Source: CAD feature listing. Evaluate the final solid. Frame: model axes, mm. Face numbers are marked on the shaded views. Coordinates: 2 decimals unless noted, no trailing zeros. Order: outer loops, then holes, each group sorted by start corner. A loop starts at its lowest first (then second) coordinate and runs counter-clockwise, first axis right, second up. Notation, with made-up numbers: (27.25, 55.25) -> (60.25, 55.25) arc R16 ccw to (60.25, 81.25) -> close; hole circle Ø10 at (-13.75, 73.25). An arc over 180 degrees is marked (long way). Write each question's results on one line, items separated by ' | '. Start each with the question number.
from build123d import *

# Parameters (mm, degrees)
IZIM1_R                     = 37.5
Y_KSEKLIK_EKSTR_ZYON1_DEPTH = 30


with BuildPart() as part:
    # Çizim1 → Yükseklik-Ekstrüzyon1 (new body)
    with BuildSketch(Plane(origin=(0, 0, 0), x_dir=(1, 0, 0), z_dir=(0, 1, 0))):
        with Locations(Location((0, 0, 0), (0, 0, 270))):
            Circle(IZIM1_R)
        with BuildLine():
            ThreePointArc((-18.874079265, -29.690864233), (-30.468569301, -17.591036688), (-35.150082319, -1.5))
            Line((-35.150082319, -1.5), (-9.196399109, -1.5))
            ThreePointArc((-9.196399109, -1.5), (-8.069561167, -4.658963312), (-5.89723766, -7.214315252))
            Line((-5.89723766, -7.214315252), (-18.874079265, -29.690864233))
        make_face(mode=Mode.SUBTRACT)
        with BuildLine():
            Line((3.299161449, -8.714315252), (16.276003054, -31.190864233))
            ThreePointArc((16.276003054, -31.190864233), (0, -35.182073376), (-16.276003054, -31.190864233))
            Line((-16.276003054, -31.190864233), (-3.299161449, -8.714315252))
            ThreePointArc((-3.299161449, -8.714315252), (0, -9.317926624), (3.299161449, -8.714315252))
        make_face(mode=Mode.SUBTRACT)
        with BuildLine():
            Line((9.196399109, -1.5), (35.150082319, -1.5))
            ThreePointArc((35.150082319, -1.5), (30.468569301, -17.591036688), (18.874079265, -29.690864233))
            Line((18.874079265, -29.690864233), (5.89723766, -7.214315252))
            ThreePointArc((5.89723766, -7.214315252), (8.069561167, -4.658963312), (9.196399109, -1.5))
        make_face(mode=Mode.SUBTRACT)
        with BuildLine():
            ThreePointArc((-35.150082319, 1.5), (-30.468569301, 17.591036688), (-18.874079265, 29.690864233))
            Line((-18.874079265, 29.690864233), (-5.89723766, 7.214315252))
            ThreePointArc((-5.89723766, 7.214315252), (-8.069561167, 4.658963312), (-9.196399109, 1.5))
            Line((-9.196399109, 1.5), (-35.150082319, 1.5))
        make_face(mode=Mode.SUBTRACT)
        with BuildLine():
            Line((6.34428877, -4), (-6.34428877, -4))
            ThreePointArc((-6.34428877, -4), (0, 7.5), (6.34428877, -4))
        make_face(mode=Mode.SUBTRACT)
        with BuildLine():
            Line((5.89723766, 7.214315252), (18.874079265, 29.690864233))
            ThreePointArc((18.874079265, 29.690864233), (30.468569301, 17.591036688), (35.150082319, 1.5))
            Line((35.150082319, 1.5), (9.196399109, 1.5))
            ThreePointArc((9.196399109, 1.5), (8.069561167, 4.658963312), (5.89723766, 7.214315252))
        make_face(mode=Mode.SUBTRACT)
        with BuildLine():
            Line((-3.299161449, 8.714315252), (-16.276003054, 31.190864233))
            ThreePointArc((-16.276003054, 31.190864233), (0, 35.182073376), (16.276003054, 31.190864233))
            Line((16.276003054, 31.190864233), (3.299161449, 8.714315252))
            ThreePointArc((3.299161449, 8.714315252), (0, 9.317926624), (-3.299161449, 8.714315252))
        make_face(mode=Mode.SUBTRACT)
    extrude(amount=Y_KSEKLIK_EKSTR_ZYON1_DEPTH)


solid = part.part
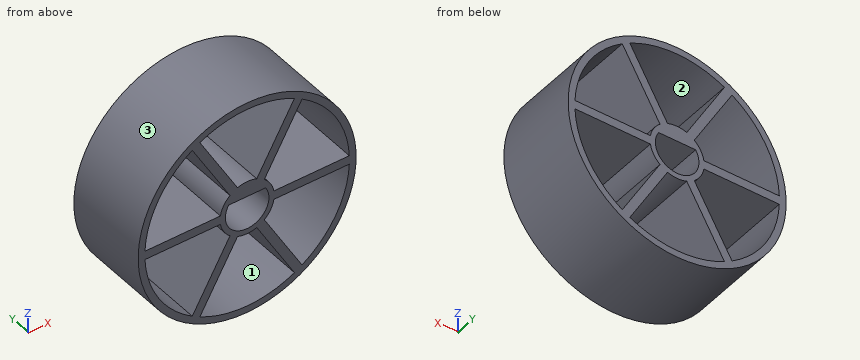
(1) First-contact query: P1, Ø1, axis at y = 19, z = -3, coming from the +X side; P2, Ø1, axis at y = 26.5, z = -24.5, coming from the +X side; P3, Ø12, axis at x = 0, z = 0, coming from the -Y side; P4, Ø8, axis at y = 7.5, z = 30, coming from the +X side. Flat tips, straight axial feed; report the tip coordinate or a pass-through.
(2) Section B-B on y = 20.5. Return the cut outline in (x, z).
(3) Draft query along X for the marked faces 1, 2 and 3. Return one class per face: released by +X, released by -X, zero draft, split by the parting line, or undercut.
(4) Section C-C on x = 0. Return the cut outline in (y, z), then the cut area to 3 significant figures.
(5) Section A-A on z = 0. Return the cut outline in (x, y).
(6) Section D-D on x = -32. Return the cut outline in (y, z), then the cut area to 3 significant figures.
(7) Line query: L1, parallel to X at y = 16, z = 0; L2, parallel to Z at x = -25, y = 20; L3, parallel to Z at x = -15, y = 18. Output: solid intervals per line, ascending.
Results list:
1) P1: stops at x = 37.42 | P2: stops at x = 28.81 | P3: stops at y = 0 | P4: stops at x = 27.02
2) outline: circle Ø75 at (0, 0); hole (-35.15, -1.5) arc R35.18 ccw to (-18.87, -29.69) -> (-5.9, -7.21) arc R9.32 cw to (-9.2, -1.5) -> close; hole (-35.15, 1.5) -> (-9.2, 1.5) arc R9.32 cw to (-5.9, 7.21) -> (-18.87, 29.69) arc R35.18 ccw to start; hole (-16.28, -31.19) arc R35.18 ccw to (16.28, -31.19) -> (3.3, -8.71) arc R9.32 cw to (-3.3, -8.71) -> close; hole (-16.28, 31.19) -> (-3.3, 8.71) arc R9.32 cw to (3.3, 8.71) -> (16.28, 31.19) arc R35.18 ccw to start; hole (-6.34, 4) arc R7.5 ccw (long way) to (6.34, 4) -> close; hole (5.9, -7.21) -> (18.87, -29.69) arc R35.18 ccw to (35.15, -1.5) -> (9.2, -1.5) arc R9.32 cw to start; hole (5.9, 7.21) arc R9.32 cw to (9.2, 1.5) -> (35.15, 1.5) arc R35.18 ccw to (18.87, 29.69) -> close
3) face 1: undercut | face 2: undercut | face 3: split by the parting line
4) outline: (0, -37.5) -> (30, -37.5) -> (30, -35.18) -> (0, -35.18) -> close; (0, -9.32) -> (30, -9.32) -> (30, -7.5) -> (0, -7.5) -> close; (0, 4) -> (30, 4) -> (30, 9.32) -> (0, 9.32) -> close; (0, 35.18) -> (30, 35.18) -> (30, 37.5) -> (0, 37.5) -> close | area: 353 mm²
5) outline: (-37.5, 0) -> (-7.5, 0) -> (-7.5, 30) -> (-37.5, 30) -> close; (7.5, 0) -> (37.5, 0) -> (37.5, 30) -> (7.5, 30) -> close
6) outline: (0, -19.55) -> (30, -19.55) -> (30, -14.62) -> (0, -14.62) -> close; (0, -1.5) -> (30, -1.5) -> (30, 1.5) -> (0, 1.5) -> close; (0, 14.62) -> (30, 14.62) -> (30, 19.55) -> (0, 19.55) -> close | area: 386 mm²
7) L1: x = -37.5 to -7.5, 7.5 to 37.5 | L2: z = -27.95 to -24.75, -1.5 to 1.5, 24.75 to 27.95 | L3: z = -34.37 to -31.82, -28.98 to -22.98, -1.5 to 1.5, 22.98 to 28.98, 31.82 to 34.37
